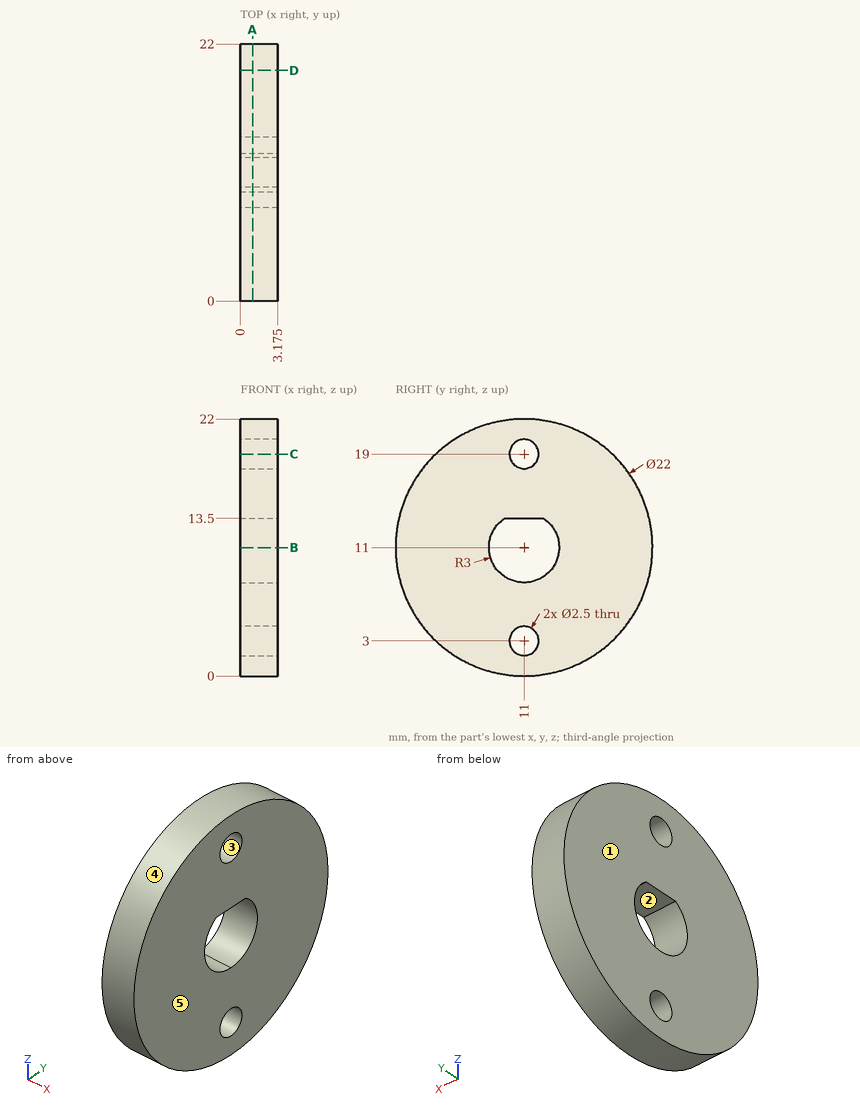
Design review of the part shown in the three views and the two pictorial views. Dimensions are in mm from the part's minimum x, y and z. A direction names the side the tool comes from. Round coordinates to 2 decimals unless told otherwise and drop trailing zeros. Write each loop counter-clockwise with the first axis right and the second up, starting at its lowest first coordinate (ties: lowest second). Pieces come first, ordered by that corner, then holes. Notation, with made-up numbers: (44, -6.75) -> (96, -6.75) arc R24 cw to (96, 16.25) -> close; hole circle Ø7 at (31, -37.5). An arc over 180 degrees is marked (long way). Use one line per item in the form item = value.
1) Take a section at A-A, the plane x = 1.05. Write out the cut boundary in (y, z).
Found:
outline = circle Ø22 at (11, 11); hole (9.34, 13.5) arc R3 ccw (long way) to (12.66, 13.5) -> close; hole circle Ø2.5 at (11, 3); hole circle Ø2.5 at (11, 19)
2) To check wall thickness, follow L1, parallel to Y at x = 0.9, z = 2.75; L2, parallel to Y at x = 1.65, z = 3; L3, parallel to Y at x = 0.3, z = 17.25. State the ranges of each line that lie inside material, in increasing order. Write a range as from..to.
Found:
L1 = 3.72..9.78, 12.22..18.28
L2 = 3.45..9.75, 12.25..18.55
L3 = 1.95..20.05
3) Take a section at D-D, the plane y = 19.75. Write out the cut boundary in (x, z) (3 decimals), and give its area (3 significant figures).
Found:
outline = (0, 4.334) -> (3.175, 4.334) -> (3.175, 17.666) -> (0, 17.666) -> close
area = 42.3 mm2
4) Tool access review of the marked faces 1 and 2: name each direction out of +Z, -Z, +X, -X, +Y, -Y from which nothing blocks a thin tool from reaching the whole face with its end or side.
Found:
face_1 = +Z, -Z, -X, +Y, -Y
face_2 = +X, -X
5) Clearance check with a flat-ended pin moving along its axis: pin 1 (2 mm diameter, centred on y = 11, z = 19, fed in from +X). State where the tip first meets the part, or that it passes through.
Found:
pin_1 = through
6) Mouldability with a two-part tool opening along Y and no side actions: class the marked faces 3, 4 and 5 as +Y half, -Y half, draft (parallel to the pull), parting line (faces both ways), or undercut.
Found:
face_3 = undercut
face_4 = parting line
face_5 = draft
7) Take a section at B-B, the plane z = 11. Write out the cut boundary in (x, y) (3 decimals).
Found:
outline = (0, 0) -> (3.175, 0) -> (3.175, 8) -> (0, 8) -> close; (0, 14) -> (3.175, 14) -> (3.175, 22) -> (0, 22) -> close
8) Take a section at C-C, the plane z = 19. Write out the cut boundary in (x, y) (3 decimals), and give its area (3 significant figures).
Found:
outline = (0, 3.45) -> (3.175, 3.45) -> (3.175, 9.75) -> (0, 9.75) -> close; (0, 12.25) -> (3.175, 12.25) -> (3.175, 18.55) -> (0, 18.55) -> close
area = 40.0 mm2
